from build123d import *

# Parameters (mm, degrees)
BOSS_EXTRUDE1_DEPTH            = 6.35
FILLET1_R                      = 1
FILLET3_R                      = 3
M2_TAPPED_HOLE1_D              = 1.6
M2_TAPPED_HOLE2_D              = 1.6
M3_CLEARANCE_HOLE1_D           = 3.4
M3_CLEARANCE_HOLE2_D           = 3.4
M3_CLEARANCE_HOLE3_D           = 3.4
M3_CLEARANCE_HOLE4_D           = 3.4
M3_TAPPED_HOLE2_D              = 2.5
M3_TAPPED_HOLE3_D              = 2.5
M3_TAPPED_HOLE4_D              = 2.5
M3_TAPPED_HOLE5_D              = 2.5
M3_TAPPED_HOLE6_D              = 2.5
M3_TAPPED_HOLE7_D              = 2.5
M3_TAPPED_HOLE8_D              = 2.5
M3_TAPPED_HOLE9_D              = 2.5
M3_TAPPED_HOLE10_D             = 2.5
M3_CLEARANCE_HOLE8_D           = 3.4
M3_CLEARANCE_HOLE7_D           = 3.4
M3_TAPPED_HOLE1_D              = 2.5
M3_CLEARANCE_HOLE6_D           = 3.4
F_25_0_25_DIAMETER_HOLE1_D     = 25
F_25_0_25_DIAMETER_HOLE1_DEPTH = 6.35
M3_CLEARANCE_HOLE5_D           = 3.4
FILLET4_R                      = 1


with BuildPart() as part:
    # Sketch1 → Boss-Extrude1 (new body)
    with BuildSketch(Plane.XY.offset(6.35)):
        Polygon((48, -56.9), (48, -52.9), (30, -52.9), (30, -48.1), (27, -48.1), (27, -49.45), (24, -49.45), (24, -48.1), (14, -48.1), (14, -44.9), (24, -44.9), (24, -43.55), (27, -43.55), (27, -44.9), (30, -44.9), (30, -28.1), (27, -28.1), (27, -29.45), (24, -29.45), (24, -28.1), (14, -28.1), (14, -24.9), (24, -24.9), (24, -23.55), (27, -23.55), (27, -24.9), (30, -24.9), (30, -20.1), (48, -20.1), (48, -16.1), (30, -16.1), (30, 28.5), (21.6, 28.5), (21.6, 25.5), (22.95, 25.5), (22.95, 22.5), (21.6, 22.5), (21.6, 18.5), (18.4, 18.5), (18.4, 22.5), (17.05, 22.5), (17.05, 25.5), (18.4, 25.5), (18.4, 28.5), (7.5, 28.5), (7.5, 34.85), (-7.5, 34.85), (-7.5, 28.5), (-18.4, 28.5), (-18.4, 25.5), (-17.05, 25.5), (-17.05, 22.5), (-18.4, 22.5), (-18.4, 18.5), (-21.6, 18.5), (-21.6, 22.5), (-22.95, 22.5), (-22.95, 25.5), (-21.6, 25.5), (-21.6, 28.5), (-30, 28.5), (-30, -16.1), (-48, -16.1), (-48, -20.1), (-30, -20.1), (-30, -24.9), (-27, -24.9), (-27, -23.55), (-24, -23.55), (-24, -24.9), (-14, -24.9), (-14, -28.1), (-24, -28.1), (-24, -29.45), (-27, -29.45), (-27, -28.1), (-30, -28.1), (-30, -44.9), (-27, -44.9), (-27, -43.55), (-24, -43.55), (-24, -44.9), (-14, -44.9), (-14, -48.1), (-24, -48.1), (-24, -49.45), (-27, -49.45), (-27, -48.1), (-30, -48.1), (-30, -52.9), (-48, -52.9), (-48, -56.9), (-30, -56.9), (-30, -80.5), (30, -80.5), (30, -56.9), align=None)
        with BuildLine():
            Line((-21.842448699, -71.75), (-21.842448699, -77.75))
            ThreePointArc((-21.842448699, -77.75), (-23.492448699, -79.4), (-25.142448699, -77.75))
            Line((-25.142448699, -77.75), (-25.142448699, -71.75))
            ThreePointArc((-25.142448699, -71.75), (-23.492448699, -70.1), (-21.842448699, -71.75))
        make_face(mode=Mode.SUBTRACT)
        with BuildLine():
            Line((21.842448699, -77.75), (21.842448699, -71.75))
            ThreePointArc((21.842448699, -71.75), (23.492448699, -70.1), (25.142448699, -71.75))
            Line((25.142448699, -71.75), (25.142448699, -77.75))
            ThreePointArc((25.142448699, -77.75), (23.492448699, -79.4), (21.842448699, -77.75))
        make_face(mode=Mode.SUBTRACT)
    extrude(amount=-BOSS_EXTRUDE1_DEPTH)

    # Fillet1
    fillet1_edges = [part.edges().sort_by_distance(p)[0] for p in [
        (-48, -56.9, 3.175),
        (-48, -52.9, 3.175),
        (-30, -48.1, 3.175),
        (-24, -48.1, 3.175),
        (-24, -44.9, 3.175),
        (-30, -44.9, 3.175),
        (-30, -28.1, 3.175),
        (-24, -28.1, 3.175),
        (-24, -24.9, 3.175),
        (-30, -24.9, 3.175),
        (-48, -20.1, 3.175),
        (-48, -16.1, 3.175),
        (48, -16.1, 3.175),
        (48, -20.1, 3.175),
        (30, -24.9, 3.175),
        (24, -24.9, 3.175),
        (24, -28.1, 3.175),
        (30, -28.1, 3.175),
        (30, -44.9, 3.175),
        (24, -44.9, 3.175),
        (24, -48.1, 3.175),
        (30, -48.1, 3.175),
        (48, -52.9, 3.175),
        (48, -56.9, 3.175),
    ]]
    fillet(fillet1_edges, radius=FILLET1_R)

    # Fillet3
    fillet3_edges = [part.edges().sort_by_distance(p)[0] for p in [
        (30, -56.9, 3.175),
        (-30, -56.9, 3.175),
        (-30, -16.1, 3.175),
        (30, -16.1, 3.175),
    ]]
    fillet(fillet3_edges, radius=FILLET3_R)

    # M2 Tapped Hole1 (through all)
    with Locations(Plane.XY.offset(6.35)):
        with Locations((-2.359287388, -35.545092005)):
            Hole(M2_TAPPED_HOLE1_D / 2)

    # M2 Tapped Hole2 (through all)
    with Locations(Plane.XY.offset(6.35)):
        with Locations((-0.7096297, -44.900765659)):
            Hole(M2_TAPPED_HOLE2_D / 2)

    # M3 Clearance Hole1 (through all)
    with Locations(Plane.XY.offset(6.35)):
        with Locations((15.5, 15.5)):
            Hole(M3_CLEARANCE_HOLE1_D / 2)

    # M3 Clearance Hole2 (through all)
    with Locations(Plane.XY.offset(6.35)):
        with Locations((-15.5, -15.5)):
            Hole(M3_CLEARANCE_HOLE2_D / 2)

    # M3 Clearance Hole3 (through all)
    with Locations(Plane.XY.offset(6.35)):
        with Locations((15.5, -15.5)):
            Hole(M3_CLEARANCE_HOLE3_D / 2)

    # M3 Clearance Hole4 (through all)
    with Locations(Plane.XY.offset(6.35)):
        with Locations((-15.5, 15.5)):
            Hole(M3_CLEARANCE_HOLE4_D / 2)

    # M3 Tapped Hole2 (through all)
    with Locations(Plane.XY.offset(6.35)):
        with Locations((23.5, -61.5)):
            Hole(M3_TAPPED_HOLE2_D / 2)

    # M3 Tapped Hole3 (through all)
    with Locations(Plane.XY.offset(6.35)):
        with Locations((23.5, -41.5)):
            Hole(M3_TAPPED_HOLE3_D / 2)

    # M3 Tapped Hole4 (through all)
    with Locations(Plane.XY.offset(6.35)):
        with Locations((23.5, -21.5)):
            Hole(M3_TAPPED_HOLE4_D / 2)

    # M3 Tapped Hole5 (through all)
    with Locations(Plane.XY.offset(6.35)):
        with Locations((23.5, -1.5)):
            Hole(M3_TAPPED_HOLE5_D / 2)

    # M3 Tapped Hole6 (through all)
    with Locations(Plane.XY.offset(6.35)):
        with Locations((-17.492448699, -71.75)):
            Hole(M3_TAPPED_HOLE6_D / 2)

    # M3 Tapped Hole7 (through all)
    with Locations(Plane.XY.offset(6.35)):
        with Locations((17.492448699, -71.75)):
            Hole(M3_TAPPED_HOLE7_D / 2)

    # M3 Tapped Hole8 (through all)
    with Locations(Plane.XY.offset(6.35)):
        with Locations((-23.5, -41.5)):
            Hole(M3_TAPPED_HOLE8_D / 2)

    # M3 Tapped Hole9 (through all)
    with Locations(Plane.XY.offset(6.35)):
        with Locations((-23.5, -61.5)):
            Hole(M3_TAPPED_HOLE9_D / 2)

    # M3 Tapped Hole10 (through all)
    with Locations(Plane.XY.offset(6.35)):
        with Locations((-23.5, -21.5)):
            Hole(M3_TAPPED_HOLE10_D / 2)

    # M3 Clearance Hole8 (through all)
    with Locations(Plane.XY.offset(6.35)):
        with Locations((-10, -46.5)):
            Hole(M3_CLEARANCE_HOLE8_D / 2)

    # M3 Clearance Hole7 (through all)
    with Locations(Plane.XY.offset(6.35)):
        with Locations((10, -46.5)):
            Hole(M3_CLEARANCE_HOLE7_D / 2)

    # M3 Tapped Hole1 (through all)
    with Locations(Plane.XY.offset(6.35)):
        with Locations((-23.5, -1.5)):
            Hole(M3_TAPPED_HOLE1_D / 2)

    # M3 Clearance Hole6 (through all)
    with Locations(Plane.XY.offset(6.35)):
        with Locations((10, -26.5)):
            Hole(M3_CLEARANCE_HOLE6_D / 2)

    # Ø25.0 (25) Diameter Hole1
    with Locations(Plane.XY.offset(6.35)):
        with Locations((0, 0)):
            Hole(F_25_0_25_DIAMETER_HOLE1_D / 2, depth=F_25_0_25_DIAMETER_HOLE1_DEPTH)

    # M3 Clearance Hole5 (through all)
    with Locations(Plane.XY.offset(6.35)):
        with Locations((-10, -26.5)):
            Hole(M3_CLEARANCE_HOLE5_D / 2)

    # Fillet4
    fillet4_edges = [part.edges().sort_by_distance(p)[0] for p in [
        (-21.6, 22.5, 3.175),
        (-18.4, 22.5, 3.175),
        (18.4, 22.5, 3.175),
        (21.6, 22.5, 3.175),
    ]]
    fillet(fillet4_edges, radius=FILLET4_R)


solid = part.part
The listing builds one solid part. Answer for the finished solid, in the listing's coordinates (mm). A direction names the side the tool comes from. Coordinates: 2 decimals unless noted, no trailing zeros. Loops run counter-clockwise (first coordinate to the right, second up) from the corner with the lowest first, then second, coordinate; pieces in that order, holes last. Notation, with made-up numbers: (36.25, 24.5) -> (47.25, 24.5) arc R6 cw to (47.25, 34.5) -> close; hole circle Ø6 at (31, -28). An arc over 180 degrees is marked (long way). Answer in a Markdown table with one row per item. Add a question column.
1. The part is cut by section A-A, the plane y = -26.5. Write down the section's boundary in (x, z), then the cut area to 3 significant figures.
2. Determine the mould class of faces 1 (the flat face through (18.4, 27, 3)), 2 (the flat face through (18, -44.9, 3)), 3 (the flat face through (-30, -36, 3)) for opening direction X: +X half, -X half, draft (parallel to the pull), parting line (faces both ways), or undercut.
3. The part is cut by section B-B, the plane x = -10. Write down the section's boundary in (y, z).
4. Consider line 1 (Y direction, x = 10, z = 4.5); line 2 (X direction, y = 0.5, z = 4.25); line 3 (Y direction, x = 40, z = 1.5). Determine where each line is inside the solid, lowest interval first. Write a range as [from, to].
5. The part is cut by section D-D, the plane y = 15.5. Write down the section's boundary in (x, z), then the cut area to 3 significant figures.
6. The part is cut by section C-C, the plane y = -1.5. Write down the section's boundary in (x, z).
7. For faces 4 (the flat face through (-30, -70, 3)), 5 (the flat face through (-14, -26, 3)), 6 (the flat face through (-21.6, 27, 3)), 7 (the flat face through (-25, -29.45, 3)), 8 (the flat face through (38, -20.1, 3)), determine the directions among +Z, -Z, +X, -X, +Y, -Y from which every point of the face is accessible in a straight line to the end or side of a thin tool.
8. Flat-ended cylindrical pins translate along their axes: P1, Ø4, axis at x = -17.49, y = -71.75, coming from the -Z side; P2, Ø1.5, axis at y = 20, z = 4.5, coming from the +X side; P3, Ø1, axis at x = -37.5, z = 1, coming from the -Y side; P4, Ø1.8, axis at y = -76, z = 4, coming from the -X side. Find the tip coordinate at first contact, or state that the pin passes through.
Answer below:
| question | item | result |
|---|---|---|
| 1 | outline | (-14, 0) -> (-11.7, 0) -> (-11.7, 6.35) -> (-14, 6.35) -> close; (-8.3, 0) -> (8.3, 0) -> (8.3, 6.35) -> (-8.3, 6.35) -> close; (11.7, 0) -> (14, 0) -> (14, 6.35) -> (11.7, 6.35) -> close |
| 1 | area | 135 mm2 |
| 2 | face 1 | undercut |
| 2 | face 2 | draft |
| 2 | face 3 | -X half |
| 3 | outline | (-80.5, 0) -> (-48.2, 0) -> (-48.2, 6.35) -> (-80.5, 6.35) -> close; (-44.8, 0) -> (-28.2, 0) -> (-28.2, 6.35) -> (-44.8, 6.35) -> close; (-24.8, 0) -> (-7.5, 0) -> (-7.5, 6.35) -> (-24.8, 6.35) -> close; (7.5, 0) -> (28.5, 0) -> (28.5, 6.35) -> (7.5, 6.35) -> close |
| 4 | line 1 | [-80.5, -48.2], [-44.8, -28.2], [-24.8, -7.5], [7.5, 28.5] |
| 4 | line 2 | [-30, -12.49], [12.49, 30] |
| 4 | line 3 | [-56.9, -52.9], [-20.1, -16.1] |
| 5 | outline | (-30, 0) -> (-17.2, 0) -> (-17.2, 6.35) -> (-30, 6.35) -> close; (-13.8, 0) -> (13.8, 0) -> (13.8, 6.35) -> (-13.8, 6.35) -> close; (17.2, 0) -> (30, 0) -> (30, 6.35) -> (17.2, 6.35) -> close |
| 5 | area | 338 mm2 |
| 6 | outline | (-30, 0) -> (-24.75, 0) -> (-24.75, 6.35) -> (-30, 6.35) -> close; (-22.25, 0) -> (-12.41, 0) -> (-12.41, 6.35) -> (-22.25, 6.35) -> close; (12.41, 0) -> (22.25, 0) -> (22.25, 6.35) -> (12.41, 6.35) -> close; (24.75, 0) -> (30, 0) -> (30, 6.35) -> (24.75, 6.35) -> close |
| 7 | face 4 | +Z, -Z, -X, -Y |
| 7 | face 5 | +Z, -Z, -X |
| 7 | face 6 | +Z, -Z, +Y |
| 7 | face 7 | +Z, -Z |
| 7 | face 8 | +Z, -Z, +X |
| 8 | P1 | z = 0 |
| 8 | P2 | x = 30 |
| 8 | P3 | y = -56.9 |
| 8 | P4 | x = -30 |
